Check sheet for the modelled part. Datum: model origin and axes. Units: mm. A direction names the side the tool comes from. Give positions to 0.01 mm unless a question says otherwise; leave off trailing zeros. Write each loop counter-clockwise with the first axis right and the second up, starting at its lowest first coordinate (ties: lowest second). Pieces come first, ordered by that corner, then holes. Notation, with made-up numbers: (17, 85.25) -> (75, 85.25) arc R21 ccw to (75, 114.25) -> close; hole circle Ø8 at (83, -26). An arc over 180 degrees is marked (long way). Use a Markdown table: item, result. Add a question column.
1. Set-up check for faces 1 (the cylindrical face through (0.54, -2.44, -2.27)), 2 (the cylindrical face through (-4.38, -8.43, -0.48)), 3 (the flat face through (2, -4, -2.5)), 4 (the cylindrical face through (4.57, -7.167, 4.437)): record each of +Z, -Z, +X, -X, +Y, -Y from which the full face is reachable in a straight line by a thin tool's end or side.
2. Cross-section at A-A (z = 5.5). Enter the section's corners in (x, y) (3 decimals).
3. Release check for a two-part mould opening along Y. For faces 5 (the flat face through (-1, 1, -1)), 6 (the flat face through (2.2, -8.4, 0)), 7 (the cylindrical face through (4.38, -8.43, 9.49)) record: released by +Y, released by -Y, zero draft, split by the parting line, or undercut.
4. Gauge pin test, flat ends, axial feed: P1, Ø1.5, axis at y = 5.5, z = 1.5, coming from the -X side; P2, Ø1.5, axis at x = -1.5, z = 3.5, coming from the -Y side; P3, Ø1.6, axis at x = -4, y = 0.5, coming from the +Z side; P4, Ø4, axis at x = 2, z = -1, coming from the +Y side. Record the tip position at first contact, or that the pin passes through.
5. Scan lines: probe 1 along X at (y, z) = (-3.5, 7); probe 2 along Y at (x, z) = (4, 6.75); probe 3 along Y at (x, z) = (0.5, 6.75). Record each from-to range of solid material in increasing order. Write a range as [from, to].
from build123d import *

# Parameters (mm, degrees)
SKETCH1_R             = 8.5
SKETCH1_R_2           = 6.5
BOSS_EXTRUDE1_DEPTH   = 9
SKETCH1_R_3           = 2.25
SKETCH1_R_4           = 0.75
BOSS_EXTRUDE1_2_DEPTH = 9
SKETCH2_R             = 9.5
BOSS_EXTRUDE2_DEPTH   = 1.5
SKETCH3_R             = 9.5
SKETCH3_R_2           = 6.5
BOSS_EXTRUDE3_DEPTH   = 1
BOSS_EXTRUDE4_REACH   = 19.051
CIRPATTERN1_COUNT     = 3
CUT_EXTRUDE2_START    = -2
SKETCH6_R             = 6.5
CUT_EXTRUDE2_DEPTH    = 2
FILLET1_R             = 3
BOSS_EXTRUDE5_START   = 1
SKETCH8_R             = 6.5
BOSS_EXTRUDE5_DEPTH   = 1
SKETCH7_R             = 1
CUT_EXTRUDE3_DEPTH    = 7
CIRPATTERN2_COUNT     = 3
FILLET2_R             = 1
SKETCH10_R            = 7
BOSS_EXTRUDE6_DEPTH   = 1
CUT_EXTRUDE5_START    = -14.5
SKETCH12_R            = 0.75
CUT_EXTRUDE5_DEPTH    = 14.5
SKETCH13_R            = 2.5
CUT_EXTRUDE6_DEPTH    = 2.5


with BuildPart() as part:
    # Sketch1 → Boss-Extrude1 (new body)
    with BuildSketch(Plane.XY):
        Circle(SKETCH1_R)
        Circle(SKETCH1_R_2, mode=Mode.SUBTRACT)
    extrude(amount=BOSS_EXTRUDE1_DEPTH)



with BuildPart() as body_2:
    # Sketch1 → Boss-Extrude1 2 (new body)
    with BuildSketch(Plane.XY):
        Circle(SKETCH1_R_3)
        Circle(SKETCH1_R_4, mode=Mode.SUBTRACT)
    extrude(amount=BOSS_EXTRUDE1_2_DEPTH)


with BuildPart() as part_1:
    add(part.part)

    add(body_2.part)  # Boss-Extrude2 merges body 2
    # Sketch2 → Boss-Extrude2 (add)
    with BuildSketch(Plane(origin=(0, 0, 0), x_dir=(-1, 0, 0), z_dir=(0, 0, -1))):
        Circle(SKETCH2_R)
    extrude(amount=BOSS_EXTRUDE2_DEPTH)

    # Sketch3 → Boss-Extrude3 (add)
    with BuildSketch(Plane.XY.offset(9)):
        Circle(SKETCH3_R)
        Circle(SKETCH3_R_2, mode=Mode.SUBTRACT)
    extrude(amount=BOSS_EXTRUDE3_DEPTH)

    # Sketch5 → Boss-Extrude4 (add, up to next)
    with BuildSketch(Plane.XY.offset(9), mode=Mode.PRIVATE) as boss_extrude4_sk1:
        with BuildLine():
            Line((2.25, 0), (6.5, 0))
            ThreePointArc((6.5, 0), (6.444391599, -0.848420249), (6.278517871, -1.682323793))
            Line((6.278517871, -1.682323793), (2.173333109, -0.582342851))
            ThreePointArc((2.173333109, -0.582342851), (2.230750938, -0.293683932), (2.25, 0))
        make_face()
    boss_extrude4_tool1 = extrude(boss_extrude4_sk1.sketch, amount=-BOSS_EXTRUDE4_REACH, mode=Mode.PRIVATE) - part_1.part
    boss_extrude4 = boss_extrude4_tool1.solids().sort_by_distance((4.665326, -0.614202, 9))[0]
    add(boss_extrude4)

    # CirPattern1: Boss-Extrude4 ×3 about axis
    cirpattern1_axis = Axis((0, 0, 0), (0, 0, 1))
    for i in range(1, CIRPATTERN1_COUNT):
        add(boss_extrude4.rotate(cirpattern1_axis, i * 360 / CIRPATTERN1_COUNT))

    # Sketch6 → Cut-Extrude2 (cut)
    with BuildSketch(Plane.XY.offset(9).offset(CUT_EXTRUDE2_START)):
        Circle(SKETCH6_R)
    extrude(amount=CUT_EXTRUDE2_DEPTH, mode=Mode.SUBTRACT)

    # Fillet1
    # the kernel refuses this fillet: 3 mm, written as the material it adds along each edge
    with BuildSketch(Plane(origin=(0, 0, 7), x_dir=(0.9659258262890711, -0.2588190451025104, 0), z_dir=(-0.2588190451025104, -0.9659258262890711, 0))) as fillet1_piece_1:
        with BuildLine():
            CenterArc((6.5 - FILLET1_R, FILLET1_R), FILLET1_R, 270, 90)
            Line((6.5 - FILLET1_R, 0), (6.5, 0))
            Line((6.5, 0), (6.5, FILLET1_R))
        make_face()
    revolve(axis=Axis((0, 0, 7), (0, 0, 1)), revolution_arc=15)
    with BuildSketch(Plane(origin=(0, 0, 7), x_dir=(-0.2588190451025142, 0.9659258262890701, 0), z_dir=(0.9659258262890701, 0.2588190451025142, 0))) as fillet1_piece_2:
        with BuildLine():
            CenterArc((6.5 - FILLET1_R, FILLET1_R), FILLET1_R, 270, 90)
            Line((6.5 - FILLET1_R, 0), (6.5, 0))
            Line((6.5, 0), (6.5, FILLET1_R))
        make_face()
    revolve(axis=Axis((0, 0, 7), (0, 0, 1)), revolution_arc=15)
    with BuildSketch(Plane(origin=(0, 0, 7), x_dir=(-0.7071067811865505, -0.7071067811865446, 0), z_dir=(-0.7071067811865446, 0.7071067811865505, 0))) as fillet1_piece_3:
        with BuildLine():
            CenterArc((6.5 - FILLET1_R, FILLET1_R), FILLET1_R, 270, 90)
            Line((6.5 - FILLET1_R, 0), (6.5, 0))
            Line((6.5, 0), (6.5, FILLET1_R))
        make_face()
    revolve(axis=Axis((0, 0, 7), (0, 0, 1)), revolution_arc=15)

    # Sketch8 → Boss-Extrude5 (add)
    with BuildSketch(Plane(origin=(0, 0, -1.5), x_dir=(-1, 0, 0), z_dir=(0, 0, -1)).offset(BOSS_EXTRUDE5_START)):
        Circle(SKETCH8_R)
    extrude(amount=-BOSS_EXTRUDE5_DEPTH)

    # Sketch7 → Cut-Extrude3 (cut)
    with BuildSketch(Plane.XY):
        with Locations((1.722075446, -4.157457896)):
            Circle(SKETCH7_R)
    cut_extrude3 = extrude(amount=-CUT_EXTRUDE3_DEPTH, mode=Mode.SUBTRACT)

    # CirPattern2: Cut-Extrude3 ×3 about axis
    cirpattern2_axis = Axis((0, 0, 0), (0, 0, 1))
    for i in range(1, CIRPATTERN2_COUNT):
        add(cut_extrude3.rotate(cirpattern2_axis, i * 360 / CIRPATTERN2_COUNT), mode=Mode.SUBTRACT)

    # Fillet2
    # the kernel refuses this fillet: 1 mm, written as the material it adds along each edge
    with BuildSketch(Plane(origin=(0, 0, 0), x_dir=(0.9268638778365579, -0.37539759184333915, 0), z_dir=(-0.37539759184333915, -0.9268638778365579, 0))) as fillet2_piece_1:
        with BuildLine():
            CenterArc((6.5 - FILLET2_R, FILLET2_R), FILLET2_R, 270, 90)
            Line((6.5 - FILLET2_R, 0), (6.5, 0))
            Line((6.5, 0), (6.5, FILLET2_R))
        make_face()
    revolve(axis=Axis((0, 0, 0), (0, 0, 1)), revolution_arc=149.097777135)
    with BuildSketch(Plane(origin=(-0.25, 0, 0), x_dir=(0, 0, 1), z_dir=(1, 0, 0))) as fillet2_piece_2_section:
        with BuildLine():
            CenterArc((FILLET2_R, -FILLET2_R), FILLET2_R, 90, 90)
            Line((0, -FILLET2_R), (0, 0))
            Line((0, 0), (FILLET2_R, 0))
        make_face()
    fillet2_piece_2 = extrude(amount=9.25, mode=Mode.PRIVATE)
    fillet2_piece_2 = fillet2_piece_2 - Plane(origin=(0, 0, 0.222961637), x_dir=(1, 0, 0), z_dir=(0, 0, -1)) * Cylinder(0.75, 23, mode=Mode.PRIVATE)
    fillet2_piece_2 = fillet2_piece_2 & Plane(origin=(0, 0, 0.222961637), x_dir=(1, 0, 0), z_dir=(0, 0, -1)) * Cylinder(8.5, 23, mode=Mode.PRIVATE)
    add(fillet2_piece_2)
    with BuildSketch(Plane(origin=(8.693332437, -2.329371406, 0), x_dir=(0, 0, 1), z_dir=(-0.9659258262890682, 0.25881904510252135, 0))) as fillet2_piece_3_section:
        with BuildLine():
            CenterArc((FILLET2_R, -FILLET2_R), FILLET2_R, 90, 90)
            Line((0, -FILLET2_R), (0, 0))
            Line((0, 0), (FILLET2_R, 0))
        make_face()
    fillet2_piece_3 = extrude(amount=9.25, mode=Mode.PRIVATE)
    fillet2_piece_3 = fillet2_piece_3 - Plane(origin=(0, 0, 0.222961624), x_dir=(1, 0, 0), z_dir=(0, 0, -1)) * Cylinder(0.75, 23, mode=Mode.PRIVATE)
    fillet2_piece_3 = fillet2_piece_3 & Plane(origin=(0, 0, 0.222961624), x_dir=(1, 0, 0), z_dir=(0, 0, -1)) * Cylinder(8.5, 23, mode=Mode.PRIVATE)
    add(fillet2_piece_3)
    with BuildSketch(Plane(origin=(0, 0, 0), x_dir=(-0.138328087862445, 0.9903864599782852, 0), z_dir=(0.9903864599782852, 0.138328087862445, 0))) as fillet2_piece_4:
        with BuildLine():
            CenterArc((6.5 - FILLET2_R, FILLET2_R), FILLET2_R, 270, 90)
            Line((6.5 - FILLET2_R, 0), (6.5, 0))
            Line((6.5, 0), (6.5, FILLET2_R))
        make_face()
    revolve(axis=Axis((0, 0, 0), (0, 0, 1)), revolution_arc=149.097777135)
    with BuildSketch(Plane(origin=(0, 0, 0), x_dir=(0.5547978045957125, 0.8319852138204006, 0), z_dir=(0.8319852138204006, -0.5547978045957125, 0))) as fillet2_piece_5:
        with BuildLine():
            CenterArc((2.25 + FILLET2_R, FILLET2_R), FILLET2_R, 180, 90)
            Line((2.25 + FILLET2_R, 0), (2.25, 0))
            Line((2.25, 0), (2.25, FILLET2_R))
        make_face()
    revolve(axis=Axis((0, 0, 0), (0, 0, 1)), revolution_arc=232.393578389)
    with BuildSketch(Plane(origin=(0.125, -0.216506351, 0), x_dir=(0, 0, 1), z_dir=(-0.49999999999999983, 0.8660254037844388, 0))) as fillet2_piece_6_section:
        with BuildLine():
            CenterArc((FILLET2_R, -FILLET2_R), FILLET2_R, 90, 90)
            Line((0, -FILLET2_R), (0, 0))
            Line((0, 0), (FILLET2_R, 0))
        make_face()
    fillet2_piece_6 = extrude(amount=9.25, mode=Mode.PRIVATE)
    fillet2_piece_6 = fillet2_piece_6 - Plane(origin=(0, 0, 0.222961635), x_dir=(1, 0, 0), z_dir=(0, 0, -1)) * Cylinder(0.75, 23, mode=Mode.PRIVATE)
    fillet2_piece_6 = fillet2_piece_6 & Plane(origin=(0, 0, 0.222961635), x_dir=(1, 0, 0), z_dir=(0, 0, -1)) * Cylinder(8.5, 23, mode=Mode.PRIVATE)
    add(fillet2_piece_6)
    with BuildSketch(Plane(origin=(-2.329371406, 8.693332437, 0), x_dir=(0, 0, 1), z_dir=(0.25881904510251996, -0.9659258262890685, 0))) as fillet2_piece_7_section:
        with BuildLine():
            CenterArc((FILLET2_R, -FILLET2_R), FILLET2_R, 90, 90)
            Line((0, -FILLET2_R), (0, 0))
            Line((0, 0), (FILLET2_R, 0))
        make_face()
    fillet2_piece_7 = extrude(amount=9.25, mode=Mode.PRIVATE)
    fillet2_piece_7 = fillet2_piece_7 - Plane(origin=(0, 0, 0.222961632), x_dir=(1, 0, 0), z_dir=(0, 0, -1)) * Cylinder(0.75, 23, mode=Mode.PRIVATE)
    fillet2_piece_7 = fillet2_piece_7 & Plane(origin=(0, 0, 0.222961632), x_dir=(1, 0, 0), z_dir=(0, 0, -1)) * Cylinder(8.5, 23, mode=Mode.PRIVATE)
    add(fillet2_piece_7)
    with BuildSketch(Plane(origin=(0, 0, 0), x_dir=(-0.7885357899741134, -0.614988868134945, 0), z_dir=(-0.614988868134945, 0.7885357899741134, 0))) as fillet2_piece_8:
        with BuildLine():
            CenterArc((6.5 - FILLET2_R, FILLET2_R), FILLET2_R, 270, 90)
            Line((6.5 - FILLET2_R, 0), (6.5, 0))
            Line((6.5, 0), (6.5, FILLET2_R))
        make_face()
    revolve(axis=Axis((0, 0, 0), (0, 0, 1)), revolution_arc=149.097777135)
    with BuildSketch(Plane(origin=(0, 0, 0), x_dir=(-0.9979192330393512, 0.06447638583352278, 0), z_dir=(0.06447638583352278, 0.9979192330393512, 0))) as fillet2_piece_9:
        with BuildLine():
            CenterArc((2.25 + FILLET2_R, FILLET2_R), FILLET2_R, 180, 90)
            Line((2.25 + FILLET2_R, 0), (2.25, 0))
            Line((2.25, 0), (2.25, FILLET2_R))
        make_face()
    revolve(axis=Axis((0, 0, 0), (0, 0, 1)), revolution_arc=232.393578389)
    with BuildSketch(Plane(origin=(0.125, 0.216506351, 0), x_dir=(0, 0, 1), z_dir=(-0.5000000000000004, -0.8660254037844384, 0))) as fillet2_piece_10_section:
        with BuildLine():
            CenterArc((FILLET2_R, -FILLET2_R), FILLET2_R, 90, 90)
            Line((0, -FILLET2_R), (0, 0))
            Line((0, 0), (FILLET2_R, 0))
        make_face()
    fillet2_piece_10 = extrude(amount=9.25, mode=Mode.PRIVATE)
    fillet2_piece_10 = fillet2_piece_10 - Plane(origin=(0, 0, 0.222961664), x_dir=(1, 0, 0), z_dir=(0, 0, -1)) * Cylinder(0.75, 23, mode=Mode.PRIVATE)
    fillet2_piece_10 = fillet2_piece_10 & Plane(origin=(0, 0, 0.222961664), x_dir=(1, 0, 0), z_dir=(0, 0, -1)) * Cylinder(8.5, 23, mode=Mode.PRIVATE)
    add(fillet2_piece_10)
    with BuildSketch(Plane(origin=(-6.363961031, -6.363961031, 0), x_dir=(0, 0, 1), z_dir=(0.7071067811865483, 0.7071067811865468, 0))) as fillet2_piece_11_section:
        with BuildLine():
            CenterArc((FILLET2_R, -FILLET2_R), FILLET2_R, 90, 90)
            Line((0, -FILLET2_R), (0, 0))
            Line((0, 0), (FILLET2_R, 0))
        make_face()
    fillet2_piece_11 = extrude(amount=9.25, mode=Mode.PRIVATE)
    fillet2_piece_11 = fillet2_piece_11 - Plane(origin=(0, 0, 0.22296162), x_dir=(1, 0, 0), z_dir=(0, 0, -1)) * Cylinder(0.75, 23, mode=Mode.PRIVATE)
    fillet2_piece_11 = fillet2_piece_11 & Plane(origin=(0, 0, 0.22296162), x_dir=(1, 0, 0), z_dir=(0, 0, -1)) * Cylinder(8.5, 23, mode=Mode.PRIVATE)
    add(fillet2_piece_11)
    with BuildSketch(Plane(origin=(0, 0, 0), x_dir=(0.44312142844363894, -0.8964615996539222, 0), z_dir=(-0.8964615996539222, -0.44312142844363894, 0))) as fillet2_piece_12:
        with BuildLine():
            CenterArc((2.25 + FILLET2_R, FILLET2_R), FILLET2_R, 180, 90)
            Line((2.25 + FILLET2_R, 0), (2.25, 0))
            Line((2.25, 0), (2.25, FILLET2_R))
        make_face()
    revolve(axis=Axis((0, 0, 0), (0, 0, 1)), revolution_arc=232.393578389)

    # Sketch10 → Boss-Extrude6 (add)
    with BuildSketch(Plane(origin=(0, 0, -2.5), x_dir=(-1, 0, 0), z_dir=(0, 0, -1))):
        Circle(SKETCH10_R)
    extrude(amount=BOSS_EXTRUDE6_DEPTH)

    # Sketch11 → Cut-Revolve1 (revolve, cut)
    with BuildSketch(Plane(origin=(0, 0, 0), x_dir=(1, 0, 0), z_dir=(0, 1, 0)), mode=Mode.PRIVATE) as cut_revolve1_sk:
        Polygon((-6.5, 2.5), (-10.5, 3.205307923), (-10.5, 0.794692077), (-6.5, 1.5), align=None)
    revolve(cut_revolve1_sk.sketch.rotate(Axis((0, 0, 0), (0, 0, -1)), 180), axis=Axis((0, 0, 0), (0, 0, -1)), mode=Mode.SUBTRACT)

    # Sketch12 → Cut-Extrude5 (cut)
    with BuildSketch(Plane.XY.offset(7).offset(CUT_EXTRUDE5_START)):
        with Locations(Location((0, 0, 0), (0, 0, 180))):
            Circle(SKETCH12_R)
    extrude(amount=CUT_EXTRUDE5_DEPTH, mode=Mode.SUBTRACT)

    # Sketch13 → Cut-Extrude6 (cut)
    with BuildSketch(Plane(origin=(0, 0, -3.5), x_dir=(-1, 0, 0), z_dir=(0, 0, -1))):
        Circle(SKETCH13_R)
    extrude(amount=-CUT_EXTRUDE6_DEPTH, mode=Mode.SUBTRACT)


solid = part_1.part
Worked answers:
| question | item | result |
|---|---|---|
| 1 | face 1 | -Z |
| 1 | face 2 | +Z, -Z |
| 1 | face 3 | +Z |
| 1 | face 4 | none |
| 2 | outline | circle Ø17 at (0, 0); hole (-4.596, -4.596) -> (-1.591, -1.591) arc R2.25 cw to (-1.125, 1.949) -> (-3.25, 5.629) arc R6.5 ccw to start; hole (-3.25, -5.629) arc R6.5 ccw to (6.279, -1.682) -> (2.173, -0.582) arc R2.25 cw to (-1.125, -1.949) -> close; hole (-1.682, 6.279) -> (-0.582, 2.173) arc R2.25 cw to (2.25, 0) -> (6.5, 0) arc R6.5 ccw to start; hole circle Ø1.5 at (0, 0) |
| 3 | face 5 | undercut |
| 3 | face 6 | zero draft |
| 3 | face 7 | split by the parting line |
| 4 | P1 | stops at x = -7.05 |
| 4 | P2 | stops at y = -8.47 |
| 4 | P3 | stops at z = 0 |
| 4 | P4 | stops at y = 9.5 |
| 5 | probe 1 | x = [-7.75, -5.48], [-3.5, -2.02], [5.48, 7.75] |
| 5 | probe 2 | y = [-7.5, -5.12], [-1.07, 0], [5.12, 7.5] |
| 5 | probe 3 | y = [-8.49, -6.48], [-2.19, -0.56], [0.56, 2.19], [6.48, 8.49] |
